from build123d import *

# Parameters (mm, degrees)
SKETCH1_R           = 7.5
SKETCH1_R_2         = 4
BOSS_EXTRUDE1_DEPTH = 12
SKETCH2_W           = 0.934125578
SKETCH2_H           = 1.3
SKETCH3_R           = 6.972941291
SKETCH3_R_2         = 4.606383091
CUT_EXTRUDE1_DEPTH  = 0.5


with BuildPart() as part:
    # Sketch1 → Boss-Extrude1 (new body, symmetric)
    with BuildSketch(Plane.XY):
        Circle(SKETCH1_R)
        Circle(SKETCH1_R_2, mode=Mode.SUBTRACT)
    extrude(amount=BOSS_EXTRUDE1_DEPTH, both=True)

    # Sketch2 → Cut-Revolve1 (revolve, cut)
    with BuildSketch(Plane(origin=(0, 0, 0), x_dir=(1, 0, 0), z_dir=(0, 1, 0))):
        with Locations((7.527516863, -8.85)):
            Rectangle(SKETCH2_W, SKETCH2_H)
        with Locations((7.527516863, 8.85)):
            Rectangle(SKETCH2_W, SKETCH2_H)
    revolve(axis=Axis((0, 0, -13.646970123), (0, 0, 1)), mode=Mode.SUBTRACT)

    # Sketch3 → Cut-Extrude1 (cut)
    with BuildSketch(Plane(origin=(0, 0, -12), x_dir=(-1, 0, 0), z_dir=(0, 0, -1))):
        Circle(SKETCH3_R)
        Circle(SKETCH3_R_2, mode=Mode.SUBTRACT)
    cut_extrude1 = extrude(amount=-CUT_EXTRUDE1_DEPTH, mode=Mode.SUBTRACT)

    # Mirror1: Cut-Extrude1 across plane
    add(cut_extrude1.mirror(Plane.XY), mode=Mode.SUBTRACT)


solid = part.part
Source: CAD feature listing. Evaluate the final solid. Frame: model axes, mm. A direction names the side the tool comes from. Round coordinates to 2 decimals unless told otherwise and drop trailing zeros. Order: outer loops, then holes, each group sorted by start corner. A loop starts at its lowest first (then second) coordinate and runs counter-clockwise, first axis right, second up. Notation, with made-up numbers: (57.5, 38) - (73.5, 38) arc R34 ccw to (73.5, 70) - close; hole circle Ø3 at (43.5, -15). An arc over 180 degrees is marked (long way). Use a Markdown table: item, result. Add a question column.
1. First-contact query: pin 1 (6.5 mm diameter, centred on x = 0, y = 0, fed in from +Z); pin 2 (3 mm diameter, centred on x = 2.5, z = -2, fed in from +Y); pin 3 (1 mm diameter, centred on y = -2.5, z = 0, fed in from -X); pin 4 (3 mm diameter, centred on y = -4, z = -2.5, fed in from -X). Flat tips, straight axial feed; report the tip coordinate or a pass-through.
2. Mould query, pull axis X, two halves, no side actions, for faces 6 (the cylindrical face through (6.734, 2.121, -8.859)), 7 (the flat face through (-1.7, 3.8, 12)), 8 (the flat face through (-1, -5, 11.5)). Classes: +X half, -X half, draft (parallel to the pull), parting line (faces both ways), or undercut.
3. Section query B-B (z = -2). Return the cut outline in (x, y), then the cut area to 3 significant figures.
4. Line query: probe 1 along Y at (x, z) = (0, 11.75); probe 2 along Z at (x, y) = (6, -4.25); probe 3 along Y at (x, z) = (0, 6.75). Output: solid intervals per line, ascending.
5. Section query A-A (x = 5.5). Return the cut outline in (y, z).
6. Section query C-C (x = -5.75). Return the cut outline in (y, z).
7. Set-up query: faces 1 (the flat face through (-6, -4, -8.2)), 2 (the cylindrical face through (-7.493, 0.33, 0.115)), 3 (the cylindrical face through (-4.394, 1.384, -11.754)), 4 (the cylindrical face through (-4.394, 1.384, 11.754)), 5 (the flat face through (-1.7, 3.8, -12)). Return all of +Z, -Z, +X, -X, +Y, -Y with unobstructed straight access to the full face (end or side cutting, diameter ignored); none if empty.
Derived:
| question | item | result |
|---|---|---|
| 1 | pin 1 | through |
| 1 | pin 2 | y = 7.43 |
| 1 | pin 3 | x = -7.23 |
| 1 | pin 4 | x = -7.07 |
| 2 | face 6 | parting line |
| 2 | face 7 | draft |
| 2 | face 8 | undercut |
| 3 | outline | circle Ø15 at (0, 0); hole circle Ø8 at (0, 0) |
| 3 | area | 126 mm2 |
| 4 | probe 1 | -7.5 to -6.97, -4.61 to -4, 4 to 4.61, 6.97 to 7.5 |
| 4 | probe 2 | -12 to -9.5, -8.2 to 8.2, 9.5 to 12 |
| 4 | probe 3 | -7.5 to -4, 4 to 7.5 |
| 5 | outline | (-5.1, -12) - (-4.29, -12) - (-4.29, -11.5) - (4.29, -11.5) - (4.29, -12) - (5.1, -12) - (5.1, -9.5) - (4.43, -9.5) - (4.43, -8.2) - (5.1, -8.2) - (5.1, 8.2) - (4.43, 8.2) - (4.43, 9.5) - (5.1, 9.5) - (5.1, 12) - (4.29, 12) - (4.29, 11.5) - (-4.29, 11.5) - (-4.29, 12) - (-5.1, 12) - (-5.1, 9.5) - (-4.43, 9.5) - (-4.43, 8.2) - (-5.1, 8.2) - (-5.1, -8.2) - (-4.43, -8.2) - (-4.43, -9.5) - (-5.1, -9.5) - close |
| 6 | outline | (-4.82, -12) - (-3.94, -12) - (-3.94, -11.5) - (3.94, -11.5) - (3.94, -12) - (4.82, -12) - (4.82, -9.5) - (4.1, -9.5) - (4.1, -8.2) - (4.82, -8.2) - (4.82, 8.2) - (4.1, 8.2) - (4.1, 9.5) - (4.82, 9.5) - (4.82, 12) - (3.94, 12) - (3.94, 11.5) - (-3.94, 11.5) - (-3.94, 12) - (-4.82, 12) - (-4.82, 9.5) - (-4.1, 9.5) - (-4.1, 8.2) - (-4.82, 8.2) - (-4.82, -8.2) - (-4.1, -8.2) - (-4.1, -9.5) - (-4.82, -9.5) - close |
| 7 | face 1 | none |
| 7 | face 2 | +Z, -Z |
| 7 | face 3 | -Z |
| 7 | face 4 | +Z |
| 7 | face 5 | -Z, +X, -X, +Y, -Y |
